Geometry: final body of the model. Coordinates: model frame, mm. Face numbers are marked on the shaded views. A direction names the side the tool comes from. Give positions to 0.01 mm unless a question says otherwise; leave off trailing zeros. Loops run counter-clockwise (first coordinate to the right, second up) from the corner with the lowest first, then second, coordinate; pieces in that order, holes last.
1. Section D-D, the plane z = -8. Output: boundary loops of the cut face in (x, y).
2. Section B-B, the plane x = -16. Output: boundary loops of the cut face in (y, z), then the cut area to 3 significant figures.
3. Section C-C, the plane y = 18.5. Output: boundary loops of the cut face in (x, z), then the cut area to 4 significant figures.
4. Material intervals for line 1 along Z through (x, y) = (-16, -26.4); line 2 along X through (y, z) = (26.5, -8); line 3 along Z through (x, y) = (-8.5, -13.5), sorted ascending.
5. Access query for the marked faces 5 and 6. Directions: +Z, -Z, +X, -X, +Y, -Y. A direction counts if a zero-diameter tool reaches every point of the face in a straight line with its end or side. Return the directions, or none.
6. Draft query along X for the marked faces 1, 2, 3 and 4. Return one class per face: +X half, -X half, draft (parallel to the pull), parting line (faces both ways), or undercut.
7. First-contact query: P1, Ø3, axis at y = -14, z = 7.5, coming from the +X side; P2, Ø6.5, axis at x = 12.37, y = 12.37, coming from the -Z side. Flat tips, straight axial feed; report the tip coordinate or a pass-through.
8. Section A-A, the plane z = 2. Output: boundary loops of the cut face in (x, y), then the cut area to 4 significant figures.
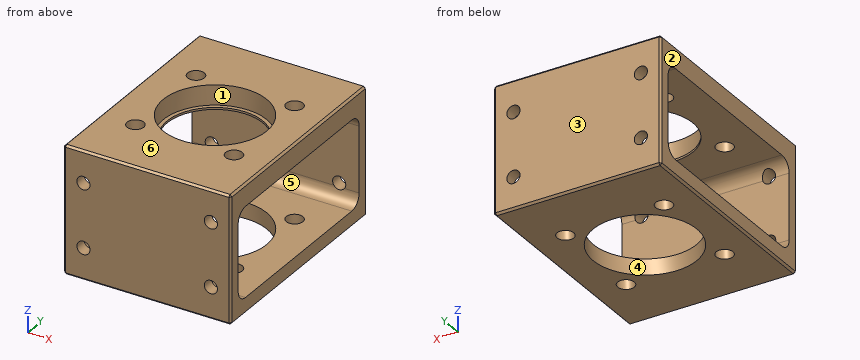
from build123d import *

# Parameters (mm, degrees)
SKETCH_1_W          = 42
SKETCH_1_H          = 32
EXTRUDE_1_DEPTH     = 27.7
SKETCH_2_R          = 13
CUT_EXTRUDE_1_DEPTH = 48.247116314
SKETCH_3_W          = 22.5
SKETCH_3_H          = 49.4
CUT_EXTRUDE_2_DEPTH = 53.79479141
SKETCH_6_R          = 2.1
CUT_EXTRUDE_4_DEPTH = 50
EXTRUDE_START       = -0.5
SKETCH_7_R          = 13
SKETCH_7_R_2        = 12
EXTRUDE_2_DEPTH     = 0.5
FILLET_2_R          = 3
SKETCH_4_R          = 1.25
CUT_EXTRUDE_3_DEPTH = 7
CHAMFER_1_SIZE      = 0.5
HOLE_WIZARD_M4_1_D  = 3.3


with BuildPart() as part:
    # 草图1 → 凸台-拉伸1 (new, symmetric)
    with BuildSketch(Plane(origin=(0, 0, 0), x_dir=(1, 0, 0), z_dir=(0, 1, 0))):
        Rectangle(SKETCH_1_W, SKETCH_1_H)
    extrude(amount=EXTRUDE_1_DEPTH, both=True)

    # 草图2 → 切除-拉伸1 (cut, through all)
    with BuildSketch(Plane.XY.offset(16)):
        Circle(SKETCH_2_R)
    extrude(amount=-CUT_EXTRUDE_1_DEPTH, mode=Mode.SUBTRACT)

    # 草图3 → 切除-拉伸2 (cut, through all)
    with BuildSketch(Plane(origin=(21, 0, 0), x_dir=(0, 0, -1), z_dir=(1, 0, 0))):
        with Locations((0.75, 0)):
            Rectangle(SKETCH_3_W, SKETCH_3_H)
    extrude(amount=-CUT_EXTRUDE_2_DEPTH, mode=Mode.SUBTRACT)

    # 草图6 → 切除-拉伸4 (cut)
    with BuildSketch(Plane.XY.offset(16)):
        with Locations((12.374368671, 12.374368671)):
            Circle(SKETCH_6_R)
        with Locations((-12.374368671, 12.374368671)):
            Circle(SKETCH_6_R)
        with Locations((12.374368671, -12.374368671)):
            Circle(SKETCH_6_R)
        with Locations((-12.374368671, -12.374368671)):
            Circle(SKETCH_6_R)
    extrude(amount=-CUT_EXTRUDE_4_DEPTH, mode=Mode.SUBTRACT)

    # 草图7 → 凸台-拉伸2 (add)
    with BuildSketch(Plane(origin=(0, 0, 10.5), x_dir=(-1, 0, 0), z_dir=(0, 0, -1)).offset(EXTRUDE_START)):
        with Locations(Location((0, 0, 0), (0, 0, 180))):
            Circle(SKETCH_7_R)
        with Locations(Location((0, 0, 0), (0, 0, 90))):
            Circle(SKETCH_7_R_2, mode=Mode.SUBTRACT)
    extrude(amount=EXTRUDE_2_DEPTH)

    # 圆角2
    fillet_2_edges = [part.edges().sort_by_distance(p)[0] for p in [
        (0, -24.7, 10.5),
        (0, 24.7, -12),
        (0, 24.7, 10.5),
        (0, -24.7, -12),
    ]]
    fillet(fillet_2_edges, radius=FILLET_2_R)

    # 草图4 → 切除-拉伸3 (cut)
    with BuildSketch(Plane(origin=(0, 27.7, 0), x_dir=(1, 0, 0), z_dir=(0, 1, 0))):
        with Locations(Location((-16, 8, 0), (0, 0, 270))):
            Circle(SKETCH_4_R)
        with Locations(Location((16, 8, 0), (0, 0, 270))):
            Circle(SKETCH_4_R)
        with Locations(Location((-16, -8, 0), (0, 0, 270))):
            Circle(SKETCH_4_R)
        with Locations(Location((16, -8, 0), (0, 0, 270))):
            Circle(SKETCH_4_R)
    cut_extrude_3 = extrude(amount=-CUT_EXTRUDE_3_DEPTH, mode=Mode.SUBTRACT)

    # 镜向1: 切除-拉伸3 across plane
    add(cut_extrude_3.mirror(Plane.ZX), mode=Mode.SUBTRACT)

    # 倒角1
    chamfer_1_edges = [part.edges().sort_by_distance(p)[0] for p in [
        (-21, 27.7, 0),
        (0, 27.7, 16),
        (21, 27.7, 0),
        (0, -27.7, 16),
        (-21, -27.7, 0),
        (0, -27.7, -16),
        (21, -27.7, 0),
        (0, 27.7, -16),
        (21, 0, 16),
        (-21, 0, 16),
        (-21, 0, -16),
        (21, 0, -16),
    ]]
    chamfer(chamfer_1_edges, length=CHAMFER_1_SIZE)

    # M4 螺纹孔1 (through all)
    with Locations(Plane(origin=(0, 27.7, 0), x_dir=(1, 0, 0), z_dir=(0, 1, 0))):
        with Locations((16, -8), (16, 8), (-16, 8), (-16, -8)):
            Hole(HOLE_WIZARD_M4_1_D / 2)


solid = part.part
Answers below:
1. outline: (-21, -27.2) - (-20.5, -27.7) - (-17.65, -27.7) - (-17.65, -24.7) - (-21, -24.7) - close; (-21, 24.7) - (-17.65, 24.7) - (-17.65, 27.7) - (-20.5, 27.7) - (-21, 27.2) - close; (-14.35, -27.7) - (14.35, -27.7) - (14.35, -24.7) - (-14.35, -24.7) - close; (-14.35, 24.7) - (14.35, 24.7) - (14.35, 27.7) - (-14.35, 27.7) - close; (17.65, -27.7) - (20.5, -27.7) - (21, -27.2) - (21, -24.7) - (17.65, -24.7) - close; (17.65, 24.7) - (21, 24.7) - (21, 27.2) - (20.5, 27.7) - (17.65, 27.7) - close
2. outline: (-27.7, -15.5) - (-27.2, -16) - (27.2, -16) - (27.7, -15.5) - (27.7, -9.65) - (24.63, -9.65) arc R3 cw to (21.7, -12) - (-21.7, -12) arc R3 cw to (-24.63, -9.65) - (-27.7, -9.65) - close; (-27.7, -6.35) - (-24.7, -6.35) - (-24.7, 6.35) - (-27.7, 6.35) - close; (-27.7, 9.65) - (-23.79, 9.65) arc R3 cw to (-21.7, 10.5) - (21.7, 10.5) arc R3 cw to (23.79, 9.65) - (27.7, 9.65) - (27.7, 15.5) - (27.2, 16) - (-27.2, 16) - (-27.7, 15.5) - close; (24.7, -6.35) - (27.7, -6.35) - (27.7, 6.35) - (24.7, 6.35) - close
2. area: 628 mm2
3. outline: (-21, -15.5) - (-20.5, -16) - (20.5, -16) - (21, -15.5) - (21, -12) - (-21, -12) - close; (-21, 10.5) - (21, 10.5) - (21, 15.5) - (20.5, 16) - (-20.5, 16) - (-21, 15.5) - close
3. area: 398.5 mm2
4. line 1: z = -16 to -9.65, -6.35 to 6.35, 9.65 to 16
4. line 2: x = -21 to -17.65, -14.35 to 14.35, 17.65 to 21
4. line 3: z = -16 to -12, 10.5 to 16
5. face 5: +X, -X
5. face 6: +Z, +X, -X, +Y, -Y
6. face 1: undercut
6. face 2: -X half
6. face 3: draft
6. face 4: undercut
7. P1: passes through
7. P2: stops at z = -16
8. outline: (-21, -27.2) - (-20.5, -27.7) - (20.5, -27.7) - (21, -27.2) - (21, -24.7) - (-21, -24.7) - close; (-21, 24.7) - (21, 24.7) - (21, 27.2) - (20.5, 27.7) - (-20.5, 27.7) - (-21, 27.2) - close
8. area: 251.5 mm2
